Input: dimensioned drawing with shaded views. Units: mm. Origin: part minimum x, y, z. Coordinates: 2 decimals unless noted, no trailing zeros. Loops run counter-clockwise (first coordinate to the right, second up) from the corner with the lowest first, then second, coordinate; pieces in that order, holes last.
(1) Mould query, pull axis X, two halves, no side actions, for the marked faces 1, 2 and 3. Classes: released by +X, released by -X, zero draft, split by the parting line, or undercut.
(2) Contact query for flat-ended pins moving along their axis: P1, Ø3.5, axis at y = 32, z = 6, coming from the +X side (1 decimal); P2, Ø6, axis at x = 24.5, z = 20.5, coming from the +Y side; P3, Ø3, axis at y = 8, z = 46, coming from the -X side (1 decimal). Output: stop coordinate, or through.
(3) Section B-B, the plane z = 26. Return loops of the section in (x, y) (1 decimal).
(4) Section A-A, the plane y = 32. Return loops of the section in (x, z) (1 decimal).
(5) Line query: L1, parallel to Y at x = 33, z = 6; L2, parallel to X at y = 15, z = 26 (1 decimal); L3, parallel to Y at x = 22.5, z = 5. Output: solid intervals per line, ascending.
(6) Section C-C, the plane x = 33. Return loops of the section in (y, z).
(7) Section D-D, the plane z = 46. Return loops of the section in (x, y) (1 decimal).
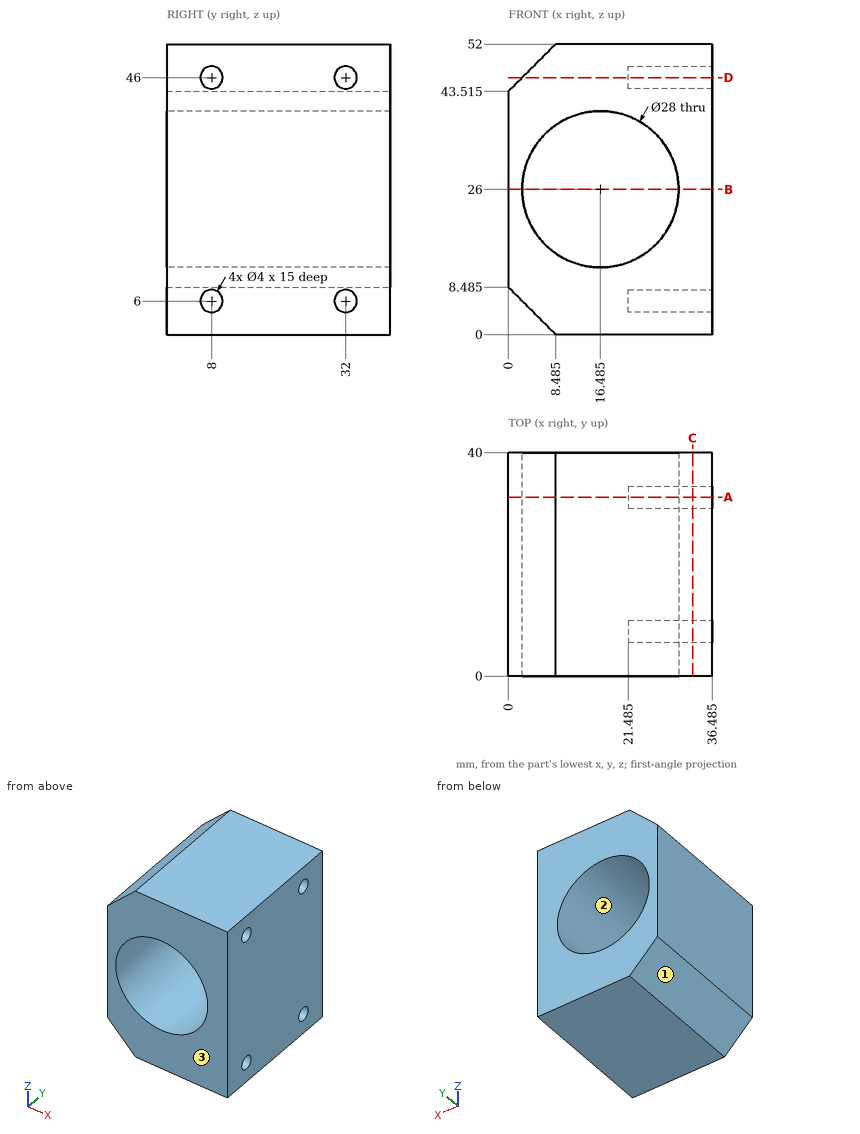
Report:
1. face 1: released by -X
1. face 2: undercut
1. face 3: zero draft
2. P1: stops at x = 21.5
2. P2: passes through
2. P3: stops at x = 1
3. outline: (0, 0) - (2.5, 0) - (2.5, 40) - (0, 40) - close; (30.5, 0) - (36.5, 0) - (36.5, 40) - (30.5, 40) - close
4. outline: (0, 8.5) - (8.5, 0) - (36.5, 0) - (36.5, 4) - (21.5, 4) - (21.5, 8) - (36.5, 8) - (36.5, 44) - (21.5, 44) - (21.5, 48) - (36.5, 48) - (36.5, 52) - (8.5, 52) - (0, 43.5) - close; hole circle Ø28 at (16.5, 26)
5. L1: y = 0 to 6, 10 to 30, 34 to 40
5. L2: x = 0 to 2.5, 30.5 to 36.5
5. L3: y = 0 to 6.27, 9.73 to 30.27, 33.73 to 40
6. outline: (0, 0) - (40, 0) - (40, 52) - (0, 52) - close; hole circle Ø4 at (8, 6); hole circle Ø4 at (8, 46); hole circle Ø4 at (32, 6); hole circle Ø4 at (32, 46)
7. outline: (2.5, 0) - (36.5, 0) - (36.5, 6) - (21.5, 6) - (21.5, 10) - (36.5, 10) - (36.5, 30) - (21.5, 30) - (21.5, 34) - (36.5, 34) - (36.5, 40) - (2.5, 40) - close
